The figure shows three views and two pictorial views of one solid part (mm, origin at its lowest corner). Answer the questions. A direction names the side the tool comes from. Coordinates: 2 decimals unless noted, no trailing zeros. Order: outer loops, then holes, each group sorted by start corner. A loop starts at its lowest first (then second) coordinate and runs counter-clockwise, first axis right, second up. Notation, with made-up numbers: M 30.25,43 L 67.25,43 A24 ccw 67.25,81 Z; hole C -17,77 d7. An arc over 180 degrees is marked long. Use a Markdown table: item, result.
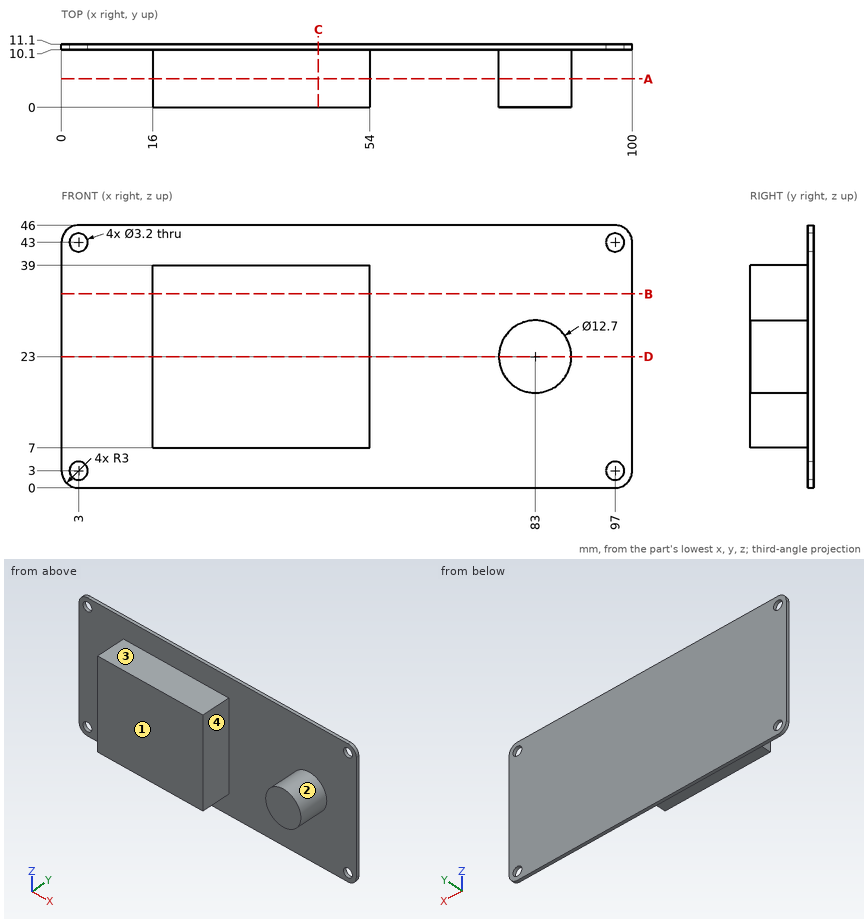
1. Section D-D on z = 23 is taken. Determine the outline of the cut face in (x, y), then the cut area to 3 significant figures.
Answers below:
| item | result |
|---|---|
| outline | M 0,10.1 L 16,10.1 L 16,0 L 54,0 L 54,10.1 L 76.65,10.1 L 76.65,0 L 89.35,0 L 89.35,10.1 L 100,10.1 L 100,11.1 L 0,11.1 Z |
| area | 612 mm² |
2. For the marked faces 1 and 2, determine the directions among +Z, -Z, +X, -X, +Y, -Y from which every point of the face is accessible in a straight line to the end or side of a thin tool.
Answers below:
| item | result |
|---|---|
| face 1 | +Z, -Z, +X, -X, -Y |
| face 2 | -Y |
3. For a pull along X with two mould halves and no side action, classify the marked faces 3 and 4 as +X half, -X half, draft (parallel to the pull), parting line (faces both ways), or undercut.
Answers below:
| item | result |
|---|---|
| face 3 | draft |
| face 4 | undercut |
4. Section C-C on x = 45 is taken. Determine the outline of the cut face in (y, z).
Answers below:
| item | result |
|---|---|
| outline | M 0,7 L 10.1,7 L 10.1,0 L 11.1,0 L 11.1,46 L 10.1,46 L 10.1,39 L 0,39 Z |
5. Section A-A on y = 5 is taken. Determine the outline of the cut face in (x, z), then the cut area to 3 significant figures.
Answers below:
| item | result |
|---|---|
| outline | M 16,7 L 54,7 L 54,39 L 16,39 Z; C 83,23 d12.7 |
| area | 1,340 mm² |
6. Section B-B on z = 34 is taken. Determine the outline of the cut face in (x, y), then the cut area to 3 significant figures.
Answers below:
| item | result |
|---|---|
| outline | M 0,10.1 L 16,10.1 L 16,0 L 54,0 L 54,10.1 L 100,10.1 L 100,11.1 L 0,11.1 Z |
| area | 484 mm² |
7. Flat-ended cylindrical pins translate along their axes: P1, Ø5, axis at x = 3, z = 43, coming from the -Y side; P2, Ø3, axis at x = 88.5, z = 19.5, coming from the -Y side; P3, Ø6, axis at y = 2.5, z = 40.5, coming from the +X side; P4, Ø5, axis at x = 82, y = 4, coming from the -Z side. Find the tip coordinate at first contact, or state that the pin passes through.
Answers below:
| item | result |
|---|---|
| P1 | y = 10.1 |
| P2 | y = 0 |
| P3 | x = 54 |
| P4 | z = 16.65 |
8. Find the intervals of material crossed by probe 1 along Z at (x, y) = (97, 10.7); probe 2 along Y at (x, z) = (7.5, 39.5); probe 3 along Z at (x, y) = (37.5, 5.5), in increasing order.
Answers below:
| item | result |
|---|---|
| probe 1 | 0 to 1.4, 4.6 to 41.4, 44.6 to 46 |
| probe 2 | 10.1 to 11.1 |
| probe 3 | 7 to 39 |
